Part model, mm, in its own coordinate system. A direction names the side the tool comes from. Round coordinates to 2 decimals unless told otherwise and drop trailing zeros. Write each loop counter-clockwise with the first axis right and the second up, starting at its lowest first coordinate (ties: lowest second). Pieces come first, ordered by that corner, then holes. Notation, with made-up numbers: M 35,62 L 42,62 A25 cw 42,79 Z; hole C 36.5,60.25 d8. An arc over 180 degrees is marked long. Use one line per item in the form item = value. Start each with the question number.
Item 1: Probe L1, parallel to Y at x = -111, z = 0.4; L2, parallel to Y at x = -95, z = 2.15; L3, parallel to X at y = 0.5, z = 4. List the from-to ranges inside material, lowest first.
Item 2: Cut at A-A, the plane x = -111.5. Give the cut face in (y, z).
Item 3: Cut at C-C, the plane y = -0.75. Give the cut face in (x, z), then the cut area to 3 significant figures.
Item 4: Flat gauge pins, fed straight in: pin 1 Ø2.5 at (x, z) = (-111, 2.5) entering from +Y; pin 2 Ø1.4 at (x, z) = (-93.5, 3) entering from -Y. Where does each tip first touch, or does it go through?
Item 5: Cut at D-D, the plane x = -101.5. Give the cut face in (y, z), then the cut area to 3 significant figures.
Item 6: Which spindle directions (+Z, -Z, +X, -X, +Y, -Y) get a long thin tool onto all of the face, cutting with end or side? Do faces 1 (the face through (-112, -4.852, 2)), 2 (the face through (-110, 1.748, 2)), 3 (the face through (-104.76, -3.34, 2.27)), 4 (the face through (-104.69, 3.22, 2.27)), 5 (the face through (-92, 4.8, 2)). Say none if no direction does.
Item 7: Mould opens along Y. For faces 6 (the face through (-103, 0, 0)), 7 (the face through (-92, -4.8, 2)), 8 (the face through (-97.88, 0.88, 2.27)) say: +Y half, -Y half, draft (parallel to the pull), parting line (faces both ways), or undercut.
Item 8: Cut at B-B, the plane y = -4. Give the cut face in (x, z), then the cut area to 3 significant figures.
from build123d import *

# Parameters (mm, degrees)
SKETCH2_R           = 4.8
SKETCH2_R_2         = 1.8
BOSS_EXTRUDE1_DEPTH = 4.6


with BuildPart() as part:
    # Sketch2 → Boss-Extrude1 (new body)
    # profile 1 of 3: a face of its own
    with BuildSketch(Plane.XY):
        with Locations((-117.224103079, -0.052328238)):
            Circle(SKETCH2_R)
        with Locations(Location((-117.224103079, -0.052328238, 0), (0, 0, 141.059939776))):
            Circle(SKETCH2_R_2, mode=Mode.SUBTRACT)
    # profile 2 of 3: a face of its own
    with BuildSketch(Plane.XY):
        with BuildLine():
            ThreePointArc((-112.774383987, -1.852328238), (-114.540821506, -4.032277987), (-117.224103079, -4.852328238))
            Line((-117.224103079, -4.852328238), (-107.224087867, -4.852328238))
            Line((-107.224087867, -4.852328238), (-102.220792221, -1.783747748))
            Line((-102.220792221, -1.783747748), (-97.224209567, -4.8))
            Line((-97.224209567, -4.8), (-87.224194355, -4.8))
            ThreePointArc((-87.224194355, -4.8), (-89.907475928, -3.979949748), (-91.673913447, -1.8))
            Line((-91.673913447, -1.8), (-96.377520534, -1.8))
            Line((-96.377520534, -1.8), (-99.335675261, -0.014271338))
            Line((-99.335675261, -0.014271338), (-96.377520534, 1.8))
            Line((-96.377520534, 1.8), (-91.673913447, 1.8))
            ThreePointArc((-91.673913447, 1.8), (-89.907475928, 3.979949748), (-87.224194355, 4.8))
            Line((-87.224194355, 4.8), (-97.224209567, 4.8))
            Line((-97.224209567, 4.8), (-102.227505213, 1.731419509))
            Line((-102.227505213, 1.731419509), (-107.224087867, 4.747671762))
            Line((-107.224087867, 4.747671762), (-117.224103079, 4.747671762))
            ThreePointArc((-117.224103079, 4.747671762), (-114.540821506, 3.92762151), (-112.774383987, 1.747671762))
            Line((-112.774383987, 1.747671762), (-108.0707769, 1.747671762))
            Line((-108.0707769, 1.747671762), (-105.112622173, -0.0380569))
            Line((-105.112622173, -0.0380569), (-108.0707769, -1.852328238))
            Line((-108.0707769, -1.852328238), (-112.774383987, -1.852328238))
        make_face()
    # profile 3 of 3: a face of its own
    with BuildSketch(Plane.XY):
        with Locations((-87.224194355, 0)):
            Circle(SKETCH2_R)
        with Locations(Location((-87.224194355, 0, 0), (0, 0, 141.059939776))):
            Circle(SKETCH2_R_2, mode=Mode.SUBTRACT)
    extrude(amount=BOSS_EXTRUDE1_DEPTH)


solid = part.part
Model answer:
q1.L1 = -4.85 to -1.85, 1.75 to 4.75
q1.L2 = -4.8 to -1.8, 1.8 to 4.8
q1.L3 = -121.99 to -118.94, -115.51 to -112.46, -106 to -98.5, -92 to -88.95, -85.5 to -82.45
q2.outline = M -4.85,0 L -1.85,0 L -1.85,4.6 L -4.85,4.6 Z; M 1.75,0 L 4.75,0 L 4.75,4.6 L 1.75,4.6 Z
q3.outline = M -121.97,0 L -118.88,0 L -118.88,4.6 L -121.97,4.6 Z; M -115.56,0 L -112.48,0 L -112.48,4.6 L -115.56,4.6 Z; M -106.27,0 L -98.12,0 L -98.12,4.6 L -106.27,4.6 Z; M -91.97,0 L -88.86,0 L -88.86,4.6 L -91.97,4.6 Z; M -85.59,0 L -82.48,0 L -82.48,4.6 L -85.59,4.6 Z
q3.area = 94.5 mm²
q4.pin_1 = 4.75
q4.pin_2 = -4.8
q5.outline = M -2.22,0 L 2.18,0 L 2.18,4.6 L -2.22,4.6 Z
q5.area = 20.2 mm²
q6.face_1 = +Z, -Z, +X, -X, -Y
q6.face_2 = +Z, -Z
q6.face_3 = +Z, -Z, -Y
q6.face_4 = +Z, -Z, +Y
q6.face_5 = +Z, -Z, +X, -X, +Y
q7.face_6 = draft
q7.face_7 = -Y half
q7.face_8 = undercut
q8.outline = M -119.95,0 L -105.83,0 L -105.83,4.6 L -119.95,4.6 Z; M -98.55,0 L -84.57,0 L -84.57,4.6 L -98.55,4.6 Z
q8.area = 129 mm²
